Geometry: final body of the model. Coordinates: model frame, mm. Face numbers are marked on the shaded views. A direction names the side the tool comes from. Coordinates: 2 decimals unless noted, no trailing zeros. Loops run counter-clockwise (first coordinate to the right, second up) from the corner with the lowest first, then second, coordinate; pieces in that order, holes last. Notation, with made-up numbers: (-25.75, 80) - (-10.75, 80) arc R16 ccw to (-10.75, 98) - close; hole circle Ø4 at (68.5, 10.25). An arc over 180 degrees is marked (long way). Return JSON: item names as keys, results as strings.
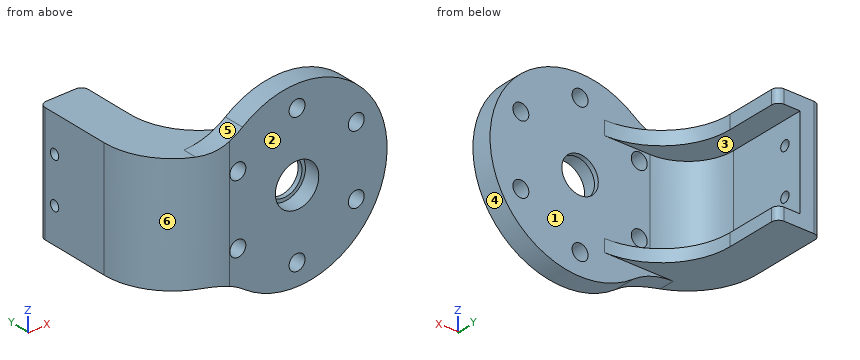
from build123d import *

# Parameters (mm, degrees)
SKETCH1_R           = 9.52
BOSS_EXTRUDE1_DEPTH = 9
BOSS_EXTRUDE2_DEPTH = 55
FILLET1_R           = 30
FILLET2_R           = 20
FILLET3_R           = 30
FILLET8_R           = 3
SKETCH3_R           = 2.2
CUT_EXTRUDE1_DEPTH  = 56
BOSS_EXTRUDE3_START = -2
SKETCH4_R           = 9.52
SKETCH4_R_2         = 8
BOSS_EXTRUDE3_DEPTH = 2
SKETCH5_R           = 3.5
CUT_EXTRUDE2_DEPTH  = 24


with BuildPart() as part:
    # Sketch1 → Boss-Extrude1 (new body)
    with BuildSketch(Plane(origin=(0, 0, 0), x_dir=(1, 0, 0), z_dir=(0, 1, 0))):
        with BuildLine():
            ThreePointArc((21.991235952, -104.520703773), (13.398585056, -99.951074742), (3.795292642, -98.372488761))
            Line((3.795292642, -98.372488761), (-13.679941451, -98.372488761))
            Line((-13.679941451, -98.372488761), (-13.679941451, -46.910148214))
            Line((-13.679941451, -46.910148214), (5.06929783, -46.910148214))
            ThreePointArc((5.06929783, -46.910148214), (14.347129848, -45.439463541), (22.715310843, -41.171603751))
            ThreePointArc((22.715310843, -41.171603751), (85.44664803, -73.567305733), (21.991235952, -104.520703773))
        make_face()
        with Locations(Location((45.949227976, -73.115853541, 0), (0, 0, 270))):
            Circle(SKETCH1_R, mode=Mode.SUBTRACT)
    extrude(amount=BOSS_EXTRUDE1_DEPTH)

    # Sketch2 → Boss-Extrude2 (add)
    with BuildSketch(Plane(origin=(0, 9, 0), x_dir=(1, 0, 0), z_dir=(0, 1, 0))):
        Polygon((-13.679941451, -46.910148214), (-4.679941451, -46.910148214), (5.320058549, -46.910148214), (5.320058549, -52.372488761), (-4.679941451, -52.372488761), (-4.679941451, -92.372488761), (5.320058549, -92.372488761), (5.320058549, -98.372488761), (-4.679941451, -98.372488761), (-13.679941451, -98.372488761), align=None)
    extrude(amount=BOSS_EXTRUDE2_DEPTH)

    # Fillet1
    fillet1_edges = [part.edges().sort_by_distance(p)[0] for p in [
        (5.320058549, 9, 95.372488761),
        (5.320058549, 9, 49.641318487),
    ]]
    fillet(fillet1_edges, radius=FILLET1_R)

    # Fillet2
    fillet2_edges = [part.edges().sort_by_distance(p)[0] for p in [
        (-4.679941451, 9, 72.372488761),
    ]]
    fillet(fillet2_edges, radius=FILLET2_R)

    # Fillet3
    fillet3_edges = [part.edges().sort_by_distance(p)[0] for p in [
        (-13.679941451, 0, 72.641318487),
    ]]
    fillet(fillet3_edges, radius=FILLET3_R)

    # Fillet8
    fillet8_edges = [part.edges().sort_by_distance(p)[0] for p in [
        (-13.679941451, 64, 72.641318487),
        (5.320058549, 64, 95.372488761),
        (5.320058549, 64, 49.641318487),
    ]]
    fillet(fillet8_edges, radius=FILLET8_R)

    # Sketch3 → Cut-Extrude1 (cut)
    with BuildSketch(Plane(origin=(-4.679941451, 0, 0), x_dir=(0, 0, -1), z_dir=(1, 0, 0))):
        with Locations((-62.372488761, 56)):
            Circle(SKETCH3_R)
        with Locations((-82.372488761, 56)):
            Circle(SKETCH3_R)
    extrude(amount=-CUT_EXTRUDE1_DEPTH, mode=Mode.SUBTRACT)

    # Sketch4 → Boss-Extrude3 (add)
    with BuildSketch(Plane(origin=(0, 9, 0), x_dir=(1, 0, 0), z_dir=(0, 1, 0)).offset(BOSS_EXTRUDE3_START)):
        with Locations(Location((45.949227976, -73.115853541, 0), (0, 0, 270))):
            Circle(SKETCH4_R)
        with Locations(Location((45.949227976, -73.115853541, 0), (0, 0, 270))):
            Circle(SKETCH4_R_2, mode=Mode.SUBTRACT)
    extrude(amount=BOSS_EXTRUDE3_DEPTH)

    # Sketch5 → Cut-Extrude2 (cut)
    with BuildSketch(Plane.XZ):
        with Locations(Location((19.968465863, 88.115853541, 0), (0, 0, 270))):
            Circle(SKETCH5_R)
        with Locations(Location((45.949227976, 103.115853541, 0), (0, 0, 270))):
            Circle(SKETCH5_R)
        with Locations(Location((71.92999009, 88.115853541, 0), (0, 0, 270))):
            Circle(SKETCH5_R)
        with Locations(Location((71.92999009, 58.115853541, 0), (0, 0, 270))):
            Circle(SKETCH5_R)
        with Locations(Location((45.949227976, 43.115853541, 0), (0, 0, 270))):
            Circle(SKETCH5_R)
        with Locations(Location((19.968465863, 58.115853541, 0), (0, 0, 270))):
            Circle(SKETCH5_R)
    extrude(amount=-CUT_EXTRUDE2_DEPTH, mode=Mode.SUBTRACT)


solid = part.part
Item 1: Section query D-D, the plane x = 62. Return loops of the section in (y, z).
Worked out:
{"outline": "(0, 37.02) - (9, 37.02) - (9, 109.21) - (0, 109.21) - close"}
Item 2: Mould query, pull axis Z, two halves, no side actions, for the marked faces 3, 4, 5 and 6. Classes: +Z half, -Z half, draft (parallel to the pull), parting line (faces both ways), or undercut.
Worked out:
{"face 3": "undercut", "face 4": "parting line", "face 5": "+Z half", "face 6": "draft"}
Item 3: Reachability of the marked faces 1 and 2 from +Z, -Z, +X, -X, +Y, -Y: full face, straight path, thin tool, end or side. Return the list, or none.
Worked out:
{"face 1": "+X, +Y", "face 2": "+Z, -Z, +X, -X, -Y"}
Item 4: Section query B-B, the plane z = 72. Return loops of the section in (x, y).
Worked out:
{"outline": "(-13.68, 30) arc R30 ccw to (16.32, 0) - (36.49, 0) - (36.49, 7) - (38.03, 7) - (38.03, 9) - (15.32, 9) arc R20 cw to (-4.68, 29) - (-4.68, 64) - (-10.68, 64) arc R3 ccw to (-13.68, 61) - close; (53.87, 7) - (55.4, 7) - (55.4, 0) - (85.43, 0) - (85.43, 9) - (53.87, 9) - close"}
Item 5: Section query C-C, the plane y = 20. Return loops of the section in (x, z), and give its area (3 significant figures).
Worked out:
{"outline": "(-11.96, 46.91) - (12.1, 46.91) - (12.1, 52.37) - (-2.54, 52.37) - (-2.54, 92.37) - (12.1, 92.37) - (12.1, 98.37) - (-11.96, 98.37) - close", "area": "653 mm^2"}
Item 6: Section query A-A, the plane y = 56. Return loops of the section in (x, z), and give its area (3 significant figures).
Worked out:
{"outline": "(-13.68, 46.91) - (5.32, 46.91) - (5.32, 52.37) - (-4.68, 52.37) - (-4.68, 60.17) - (-13.68, 60.17) - close; (-13.68, 64.57) - (-4.68, 64.57) - (-4.68, 80.17) - (-13.68, 80.17) - close; (-13.68, 84.57) - (-4.68, 84.57) - (-4.68, 92.37) - (5.32, 92.37) - (5.32, 98.37) - (-13.68, 98.37) - close", "area": "499 mm^2"}
Item 7: Ray query, probe 1 along Z at (x, y) = (-3, 51.5); probe 2 along Y at (x, z) = (33.5, 68); probe 3 along X at (y, z) = (32, 85.5). Return the intervals inside material, ascending. Write a range as from..to.
Worked out:
{"probe 1": "46.91..52.37, 92.37..98.37", "probe 2": "0..9", "probe 3": "-13.68..-4.68"}
Item 8: First-contact query: pin 1 Ø10 at (x, z) = (63, 104.5) entering from +Y; pin 2 Ø6 at (y, z) = (46, 48.5) entering from +X; pin 3 Ø20 at (x, y) = (8.5, 46) entering from -Z. Flat tips, straight axial feed; report the tip coordinate or a pass-through.
Worked out:
{"pin 1": "y = 9", "pin 2": "x = 5.32", "pin 3": "z = 46.91"}
